For this review, take the finished solid that the model builds, in its own axes (mm). A direction names the side the tool comes from. Coordinates: 2 decimals unless noted, no trailing zeros. Write each loop counter-clockwise with the first axis right and the second up, starting at its lowest first coordinate (ties: lowest second). Pieces come first, ordered by that corner, then holes. Notation, with made-up numbers: M -25.5,33 L -4.5,33 A11 cw -4.5,51 Z; hole C 49.5,-19.5 d2. An arc over 180 degrees is marked long. Return JSON: item names as keys, results as strings.
```python
from build123d import *

# Parameters (mm, degrees)
SKETCH1_R                = 31.75
BOSS_EXTRUDE1_DEPTH      = 24.13
SKETCH2_R                = 20.828
BOSS_EXTRUDE2_DEPTH      = 24.13
SKETCH3_R                = 8.7249
BOSS_EXTRUDE3_DEPTH      = 35.56
BOSS_EXTRUDE3_DEPTH_BACK = 1.27
SKETCH4_R                = 16.51
BOSS_EXTRUDE4_DEPTH      = 5.08
SKETCH5_R                = 19.05
BOSS_EXTRUDE5_DEPTH      = 56.896
SKETCH6_W                = 20.066
SKETCH6_H                = 27.432
BOSS_EXTRUDE6_DEPTH      = 17.399
SKETCH7_W                = 22.86
SKETCH7_H                = 22.0218
BOSS_EXTRUDE7_DEPTH      = 20.32
SKETCH8_W                = 27.051
SKETCH8_H                = 22.0218
BOSS_EXTRUDE8_DEPTH      = 10.414
SKETCH9_W                = 16.51
SKETCH9_H                = 20.32
BOSS_EXTRUDE9_DEPTH      = 18.542
SKETCH10_W               = 13.208
SKETCH10_H               = 13.716
CUT_EXTRUDE1_DEPTH       = 18.542
BOSS_EXTRUDE10_START     = -6.35
BOSS_EXTRUDE10_DEPTH     = 17.78
BOSS_EXTRUDE11_DEPTH     = 15.24
SKETCH13_W               = 17.847333413
SKETCH13_H               = 6.050107252
BOSS_EXTRUDE12_DEPTH     = 15.24
SKETCH14_R               = 3.683
BOSS_EXTRUDE13_DEPTH     = 17.78
SKETCH15_R               = 3.683
CUT_EXTRUDE2_DEPTH       = 117.691841319
SKETCH16_R               = 4
BOSS_EXTRUDE14_DEPTH     = 17.78
SKETCH17_R               = 4
BOSS_EXTRUDE15_DEPTH     = 12


with BuildPart() as part:
    # Sketch1 → Boss-Extrude1 (new body)
    with BuildSketch(Plane(origin=(0, 0, 0), x_dir=(1, 0, 0), z_dir=(0, 1, 0))):
        with Locations(Location((0, 0, 0), (0, 0, 90))):
            Circle(SKETCH1_R)
    extrude(amount=BOSS_EXTRUDE1_DEPTH)

    # Sketch2 → Boss-Extrude2 (add)
    with BuildSketch(Plane(origin=(0, 24.13, 0), x_dir=(1, 0, 0), z_dir=(0, 1, 0))):
        with Locations((14.775728205, -34.29)):
            Circle(SKETCH2_R)
    extrude(amount=-BOSS_EXTRUDE2_DEPTH)

    # Sketch3 → Boss-Extrude3 (add, two sides)
    with BuildSketch(Plane(origin=(0, 0, 0), x_dir=(0, 0, -1), z_dir=(1, 0, 0))) as boss_extrude3_sk:
        with Locations((-60.96, 17.8435)):
            Circle(SKETCH3_R)
    extrude(amount=BOSS_EXTRUDE3_DEPTH)
    extrude(boss_extrude3_sk.sketch, amount=-BOSS_EXTRUDE3_DEPTH_BACK)

    # Sketch4 → Boss-Extrude4 (add)
    with BuildSketch(Plane.ZY.offset(1.27)):
        with Locations(Location((60.96, 17.8435, 0), (0, 0, 157.618661281))):
            Circle(SKETCH4_R)
    extrude(amount=BOSS_EXTRUDE4_DEPTH)

    # Sketch5 → Boss-Extrude5 (add)
    with BuildSketch(Plane.ZY.offset(6.35)):
        with Locations((60.96, 17.8435)):
            Circle(SKETCH5_R)
    extrude(amount=BOSS_EXTRUDE5_DEPTH)

    # Sketch6 → Boss-Extrude6 (add)
    with BuildSketch(Plane.ZY.offset(63.246)):
        with Locations((60.96, 17.8435)):
            Rectangle(SKETCH6_W, SKETCH6_H)
    extrude(amount=BOSS_EXTRUDE6_DEPTH)

    # Sketch7 → Boss-Extrude7 (add)
    with BuildSketch(Plane(origin=(0, 0, 50.927), x_dir=(-1, 0, 0), z_dir=(0, 0, -1))):
        with Locations((65.4558, 17.8435)):
            Rectangle(SKETCH7_W, SKETCH7_H)
    extrude(amount=BOSS_EXTRUDE7_DEPTH)

    # Sketch8 → Boss-Extrude8 (add)
    with BuildSketch(Plane(origin=(0, 0, 30.607), x_dir=(-1, 0, 0), z_dir=(0, 0, -1))):
        with Locations((67.5513, 17.8435)):
            Rectangle(SKETCH8_W, SKETCH8_H)
    extrude(amount=BOSS_EXTRUDE8_DEPTH)

    # Sketch9 → Boss-Extrude9 (add)
    with BuildSketch(Plane(origin=(0, 0, 20.193), x_dir=(-1, 0, 0), z_dir=(0, 0, -1))):
        with Locations((69.7738, 18.6944)):
            Rectangle(SKETCH9_W, SKETCH9_H)
    extrude(amount=BOSS_EXTRUDE9_DEPTH)

    # Sketch10 → Cut-Extrude1 (cut)
    with BuildSketch(Plane(origin=(0, 0, 1.651), x_dir=(-1, 0, 0), z_dir=(0, 0, -1))):
        with Locations((69.977, 16.8402)):
            Rectangle(SKETCH10_W, SKETCH10_H)
    extrude(amount=-CUT_EXTRUDE1_DEPTH, mode=Mode.SUBTRACT)

    # Sketch11 → Boss-Extrude10 (add)
    with BuildSketch(Plane.XZ.offset(BOSS_EXTRUDE10_START)):
        with BuildLine():
            Line((-31.398919365, -4.708541462), (-54.0258, 26.543))
            Line((-54.0258, 26.543), (-54.0258, 40.386))
            Line((-54.0258, 40.386), (-5.140204311, 40.386))
            ThreePointArc((-5.140204311, 40.386), (-5.994749346, 35.836882769), (-5.823485644, 31.211368361))
            ThreePointArc((-5.823485644, 31.211368361), (-25.863813313, 18.415364805), (-31.398919365, -4.708541462))
        make_face()
    extrude(amount=-BOSS_EXTRUDE10_DEPTH)

    # Sketch12 → Boss-Extrude11 (add)
    with BuildSketch(Plane(origin=(0, 24.13, 0), x_dir=(1, 0, 0), z_dir=(0, 1, 0))):
        with BuildLine():
            Line((35.60368127, -34.334216844), (35.56, -54.909892748))
            Line((35.56, -54.909892748), (17.712666587, -54.909892748))
            ThreePointArc((17.712666587, -54.909892748), (30.492983885, -47.956508622), (35.60368127, -34.334216844))
        make_face()
    extrude(amount=-BOSS_EXTRUDE11_DEPTH)

    # Sketch13 → Boss-Extrude12 (add)
    with BuildSketch(Plane.XZ.offset(-8.89)):
        with Locations((26.636333294, 57.934946374)):
            Rectangle(SKETCH13_W, SKETCH13_H)
    extrude(amount=-BOSS_EXTRUDE12_DEPTH)

    # Sketch14 → Boss-Extrude13 (add)
    with BuildSketch(Plane(origin=(0, 24.13, 0), x_dir=(1, 0, 0), z_dir=(0, 1, 0))):
        with BuildLine():
            Line((-26.194044188, 17.942534634), (-21.621621656, 43.757348716))
            ThreePointArc((-21.621621656, 43.757348716), (-17.617871268, 48.521350377), (-11.490249612, 47.436001661))
            Line((-11.490249612, 47.436001661), (8.579823912, 30.568760551))
            ThreePointArc((8.579823912, 30.568760551), (-10.836077898, 29.843624374), (-26.194044188, 17.942534634))
        make_face()
        with Locations(Location((-15.494, 42.672, 0), (0, 0, 270))):
            Circle(SKETCH14_R, mode=Mode.SUBTRACT)
        with BuildLine():
            Line((46.054149639, 13.727593162), (22.766210397, 22.130570805))
            ThreePointArc((22.766210397, 22.130570805), (31.252220413, 5.60010886), (29.034123834, -12.848429989))
            Line((29.034123834, -12.848429989), (47.955285562, 3.118028175))
            ThreePointArc((47.955285562, 3.118028175), (50.067435201, 8.971621337), (46.054149639, 13.727593162))
        make_face()
        with Locations(Location((43.942, 7.874, 0), (0, 0, 270))):
            Circle(SKETCH14_R, mode=Mode.SUBTRACT)
    extrude(amount=-BOSS_EXTRUDE13_DEPTH)

    # Sketch15 → Cut-Extrude2 (cut, through all)
    with BuildSketch(Plane(origin=(0, 24.13, 0), x_dir=(1, 0, 0), z_dir=(0, 1, 0))):
        with Locations(Location((-31.242, -22.86, 0), (0, 0, 270))):
            Circle(SKETCH15_R)
        with Locations(Location((43.942, 7.874, 0), (0, 0, 270))):
            Circle(SKETCH15_R)
        with Locations(Location((-15.494, 42.672, 0), (0, 0, 270))):
            Circle(SKETCH15_R)
    extrude(amount=-CUT_EXTRUDE2_DEPTH, mode=Mode.SUBTRACT)

    # Sketch16 → Boss-Extrude14 (add)
    with BuildSketch(Plane(origin=(0, 24.13, 0), x_dir=(1, 0, 0), z_dir=(0, 1, 0))):
        with Locations(Location((0, 0, 0), (0, 0, 270))):
            Circle(SKETCH16_R)
    extrude(amount=BOSS_EXTRUDE14_DEPTH)

    # Sketch17 → Boss-Extrude15 (add)
    with BuildSketch(Plane(origin=(0, 24.13, 0), x_dir=(1, 0, 0), z_dir=(0, 1, 0))):
        with BuildLine():
            Line((-2.899494937, -7), (-0.949747468, -8.949747468))
            ThreePointArc((-0.949747468, -8.949747468), (0, -9), (0.949747468, -8.949747468))
            Line((0.949747468, -8.949747468), (2.899494937, -7))
            Line((2.899494937, -7), (5.656854249, -7))
            ThreePointArc((5.656854249, -7), (6.363961031, -6.363961031), (7, -5.656854249))
            Line((7, -5.656854249), (7, -2.899494937))
            Line((7, -2.899494937), (8.949747468, -0.949747468))
            ThreePointArc((8.949747468, -0.949747468), (9, 0), (8.949747468, 0.949747468))
            Line((8.949747468, 0.949747468), (7, 2.899494937))
            Line((7, 2.899494937), (7, 5.656854249))
            ThreePointArc((7, 5.656854249), (6.363961031, 6.363961031), (5.656854249, 7))
            Line((5.656854249, 7), (2.899494937, 7))
            Line((2.899494937, 7), (0.949747468, 8.949747468))
            ThreePointArc((0.949747468, 8.949747468), (0, 9), (-0.949747468, 8.949747468))
            Line((-0.949747468, 8.949747468), (-2.899494937, 7))
            Line((-2.899494937, 7), (-5.656854249, 7))
            ThreePointArc((-5.656854249, 7), (-6.363961031, 6.363961031), (-7, 5.656854249))
            Line((-7, 5.656854249), (-7, 2.899494937))
            Line((-7, 2.899494937), (-8.949747468, 0.949747468))
            ThreePointArc((-8.949747468, 0.949747468), (-9, 0), (-8.949747468, -0.949747468))
            Line((-8.949747468, -0.949747468), (-7, -2.899494937))
            Line((-7, -2.899494937), (-7, -5.656854249))
            ThreePointArc((-7, -5.656854249), (-6.363961031, -6.363961031), (-5.656854249, -7))
            Line((-5.656854249, -7), (-2.899494937, -7))
        make_face()
        with Locations(Location((0, 0, 0), (0, 0, 270))):
            Circle(SKETCH17_R, mode=Mode.SUBTRACT)
    extrude(amount=BOSS_EXTRUDE15_DEPTH)


solid = part.part
```
1. We need section B-B (x = -65.5). State the section outline as (y, z) points.
Checks:
{"outline": "M 4.13,50.93 L 6.83,50.93 L 6.83,20.19 L 8.53,20.19 L 8.53,1.65 L 9.98,1.65 L 9.98,20.19 L 23.7,20.19 L 23.7,1.65 L 28.85,1.65 L 28.85,50.93 L 31.56,50.93 L 31.56,70.99 L 4.13,70.99 Z"}
2. We need section A-A (z = 22.86). State the section outline as (x, y) points (3 decimals), plus the area to 3 significant figures.
Checks:
{"outline": "M -81.077,6.833 L -54.026,6.833 L -54.026,28.854 L -81.077,28.854 Z; M -51.359,6.35 L -34.925,6.35 L -34.925,24.13 L -51.359,24.13 Z; M -27.559,6.35 L -22.034,6.35 L -22.034,0 L 32.187,0 L 32.187,24.13 L -27.559,24.13 Z", "area": "2,290 mm2"}
3. We need section D-D (y = 38.5). State the section outline as (x, z) points.
Checks:
{"outline": "C 0,0 d8"}
4. For faces 1 (the face through (2, 36.13, 4)), 2 (the face through (-67, 28.854, 27)), 3 (the face through (-70, 17, 20.193)), 4 (the face through (-30, 15, 40.386)), list the 3-axis set-ups (+Z, -Z, +X, -X, +Y, -Y) from which the entire face can be reached by the end or side of a thin tool; tool diameter is ignored.
Checks:
{"face 1": "+Y", "face 2": "-Z, -X, +Y", "face 3": "-Z", "face 4": "+Y, -Y"}
5. Wall thickness on L1, parallel to Y at x = -70, z = 2; L2, parallel to Y at x = 17, z = -23; L3, parallel to X at y = 22.5, z = 21.5: over which ranges is each line inside the solid? List them lowest first. Write a range as from..to.
Checks:
{"L1": "8.53..9.98, 23.7..28.85", "L2": "0..24.13", "L3": "-81.08..-54.03, -50.37..-34.66, -27.82..31.21"}
6. Clearance check with flat-ended pins moving along their axes: pin 1 Ø6 at (x, y) = (16, 18.5) entering from -Z; pin 2 Ø4 at (x, z) = (-68.5, 9.5) entering from +Y; pin 3 Ø8 at (y, z) = (23.5, -6.5) entering from -X. State where each tip first meets the part, or that it passes through.
Checks:
{"pin 1": "z = -28.97", "pin 2": "y = 28.85", "pin 3": "x = -33"}
7. Draft analysis for pull direction X (two halves, no side actions). For faces 5 (the face through (-80.645, 18, 61)), 6 (the face through (-61.519, 19, 11)), 7 (the face through (29, 8.89, 53)), state which applies: +X half, -X half, draft (parallel to the pull), parting line (faces both ways), or undercut.
Checks:
{"face 5": "-X half", "face 6": "undercut", "face 7": "draft"}
